Input: dimensioned drawing with shaded views. Units: mm. Origin: part minimum x, y, z. A direction names the side the tool comes from. Round coordinates to 2 decimals unless told otherwise and drop trailing zeros. Write each loop counter-clockwise with the first axis right and the second up, starting at its lowest first coordinate (ties: lowest second). Pieces come first, ordered by that corner, then holes. Notation, with made-up numbers: M 5,-13 L 18,-13 A20 cw 18,-3 Z; hole C 75.25,26 d6. An arc over 180 degrees is marked long. Answer as CSV lines item,"result". Start each with the question number.
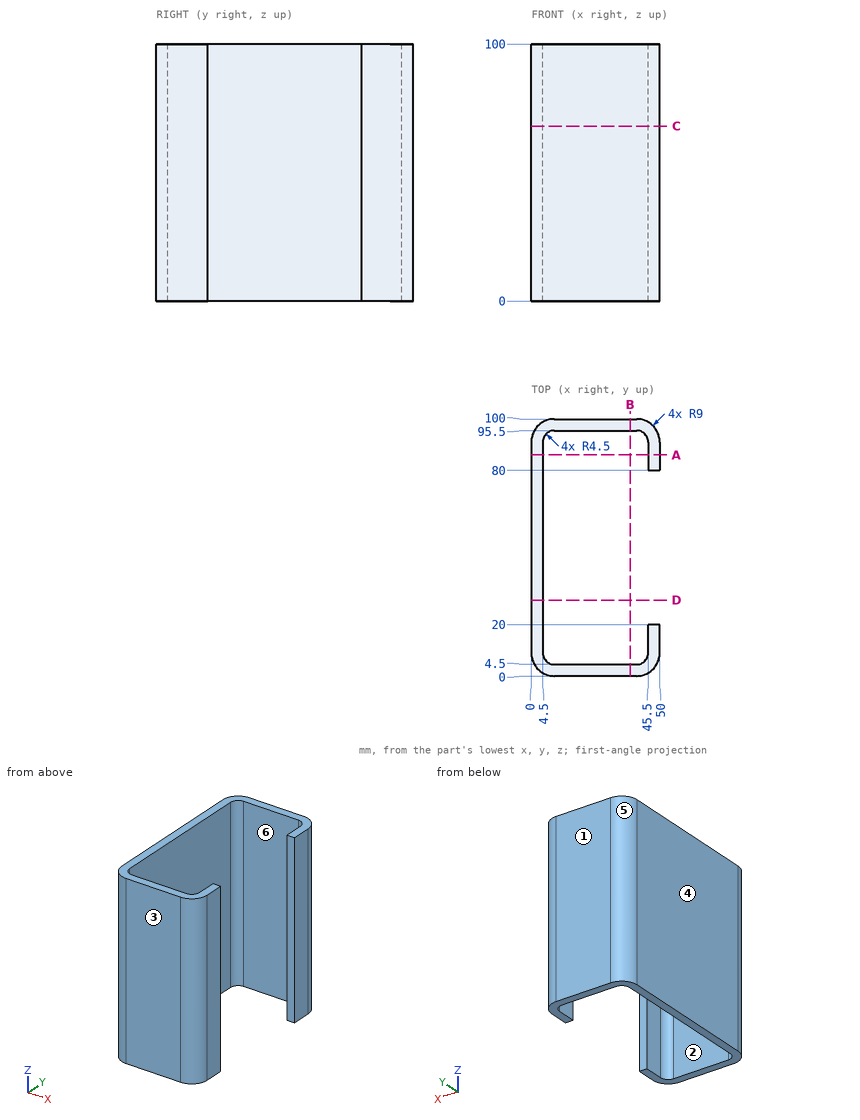
Item 1: Access query for the marked faces 5 and 6. Directions: +Z, -Z, +X, -X, +Y, -Y. A direction counts if a zero-diameter tool reaches every point of the face in a straight line with its end or side. Return the directions, or none.
Item 2: Line query: line 1 (Y direction, x = 28, z = 83.5); line 2 (X direction, y = 91.5, z = 62.5); line 3 (X direction, y = 78, z = 41). Output: solid intervals per line, ascending. Write a range as [from, to].
Item 3: Cut plane B-B, the plane x = 38.5. Return loops of the section in (y, z), plus the area to 3 significant figures.
Item 4: Cut plane A-A, the plane y = 86. Return loops of the section in (x, z), plus the area to 3 significant figures.
Item 5: Cut plane D-D, the plane y = 29.5. Return loops of the section in (x, z).
Item 6: Draft query along Y for the marked faces 1, 2, 3 and 4. Return one class per face: +Y half, -Y half, draft (parallel to the pull), parting line (faces both ways), or undercut.
Item 7: Pin query (flat end, axial travel): pin 1 Ø3.5 at (x, z) = (47.5, 37.5) entering from +Y; pin 2 Ø3.5 at (x, z) = (47, 66) entering from -Y. Return the tip coordinate at first contact, or that it passes through.
Item 8: Cut plane C-C, the plane z = 68. Return loops of the section in (x, y).
Results list:
1,face 5,"+Z, -Z, -X, +Y"
1,face 6,"+Z, -Z"
2,line 1,"[0, 4.5], [95.5, 100]"
2,line 2,"[0.01, 4.53], [45.47, 49.99]"
2,line 3,"[0, 4.5]"
3,outline,"M 0,0 L 4.5,0 L 4.5,100 L 0,100 Z; M 95.5,0 L 100,0 L 100,100 L 95.5,100 Z"
3,area,"900 mm²"
4,outline,"M 0,0 L 4.5,0 L 4.5,100 L 0,100 Z; M 45.5,0 L 50,0 L 50,100 L 45.5,100 Z"
4,area,"900 mm²"
5,outline,"M 0,0 L 4.5,0 L 4.5,100 L 0,100 Z"
6,face 1,"+Y half"
6,face 2,"undercut"
6,face 3,"-Y half"
6,face 4,"draft"
7,pin 1,"y = 98.64"
7,pin 2,"y = 1.07"
8,outline,"M 0,9 A9 ccw 9,0 L 41,0 A9 ccw 50,9 L 50,20 L 45.5,20 L 45.5,9 A4.5 cw 41,4.5 L 9,4.5 A4.5 cw 4.5,9 L 4.5,91 A4.5 cw 9,95.5 L 41,95.5 A4.5 cw 45.5,91 L 45.5,80 L 50,80 L 50,91 A9 ccw 41,100 L 9,100 A9 ccw 0,91 Z"
